```python
from build123d import *

# Parameters (mm, degrees)
F0_W     = 5.0226673484
F0_H     = 50.8
F2_R     = 5.08
F4_W     = 74.5882093906
F4_H     = 114.3385246396
F5_DEPTH = 21.6480400413


with BuildPart() as f1:
    # F0 (on Front) → F1 (revolve)
    with BuildSketch(Plane.XZ):
        Polygon((0, -25.4), (0, 0), (-5.0226673484, 0), (-25.4, 0), align=None)
        with Locations((-2.5113336742, 25.4)):
            Rectangle(F0_W, F0_H)
    revolve(axis=Axis((0, 0, 25.4), (0, 0, 1)))

    # F2
    f2_edges = [f1.edges().sort_by_distance(p)[0] for p in [
        (25.4, 0, 0),
    ]]
    fillet(f2_edges, radius=F2_R)

    # F4 (on offset) → F5 (cut)
    with BuildSketch(Plane.XY.offset(52.3276198655)):
        with Locations((8.5238665342, 15.934009105)):
            Rectangle(F4_W, F4_H)
    extrude(amount=-F5_DEPTH, mode=Mode.SUBTRACT)


solid = f1.part
```
Can you work these out from the model? Positions are in its coordinate system, mm. A direction names the side the tool comes from. Give positions to 0.01 mm unless a question says otherwise; leave off trailing zeros. Order: outer loops, then holes, each group sorted by start corner. A loop starts at its lowest first (then second) coordinate and runs counter-clockwise, first axis right, second up. Notation, with made-up numbers: M 43.5,20.5 L 55.5,20.5 A19 cw 55.5,44.5 Z; hole C 22.5,79 d5. An arc over 180 degrees is marked long. Write item = value, one per line. Start each with the question number.
Q1. I need wall thicknesses on probe 1 along Y at (x, z) = (0, 21.5); probe 2 along Y at (x, z) = (-2, -5); probe 3 along X at (y, z) = (-1.5, -2). Which ranges of each line are inside material? Lowest first, please. Write a range as [from, to].
Q2. Will these pins go through, and if not, where does the flat tip stop? pin 1 Ø1 at (x, z) = (10, -7) entering from +Y; pin 2 Ø12 at (x, z) = (-1.5, -9) entering from -Y; pin 3 Ø4 at (y, z) = (6.5, 21) entering from +X.
Q3. Suppose I cut it at A-A (z = -9.5). Write out the boundary of the cut face in (x, y).
Q4. For faces 1 (the flat face through (0, 0, 30.68)), 2 (the cylindrical face through (3.986, 3.056, 15.555)), which set-ups out of +Z, -Z, +X, -X, +Y, -Y let a thin tool reach every point of the face, with its end or its side?
Check result:
q1.probe_1 = [-5.02, 5.02]
q1.probe_2 = [-18.11, 18.11]
q1.probe_3 = [-17.11, 17.11]
q2.pin_1 = 15.17
q2.pin_2 = -18.22
q2.pin_3 = 2.23
q3.outline = C 0,0 d31.8
q4.face_1 = +Z, +X, -X, +Y, -Y
q4.face_2 = +Z
